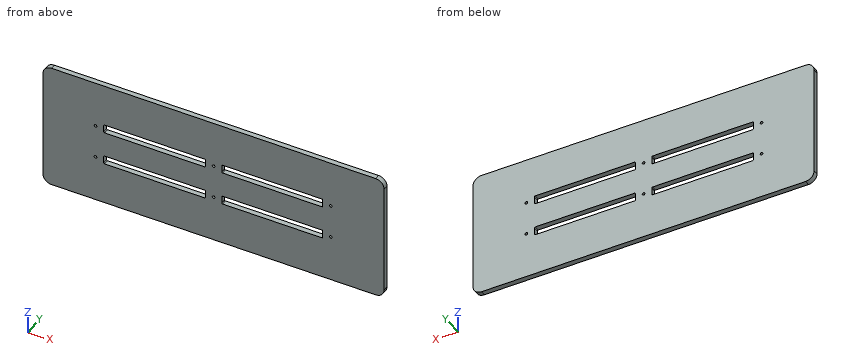
from build123d import *

# Parameters (mm, degrees)
IZIM1_W                     = 400
IZIM1_H                     = 150
IZIM1_W_2                   = 119.18
IZIM1_H_2                   = 10
IZIM1_W_3                   = 118.39
Y_KSEKLIK_EKSTR_ZYON1_DEPTH = 6
RADYUS1_R                   = 10
RADYUS2_R                   = 1
IZIM2_R                     = 1.575
KES_EKSTR_ZYON1_DEPTH       = 7


with BuildPart() as part:
    # Çizim1 → Yükseklik-Ekstrüzyon1 (new body)
    with BuildSketch(Plane(origin=(0, 0, 0), x_dir=(1, 0, 0), z_dir=(0, 1, 0))):
        Rectangle(IZIM1_W, IZIM1_H)
        with Locations((-69.19, 20)):
            Rectangle(IZIM1_W_2, IZIM1_H_2, mode=Mode.SUBTRACT)
        with Locations((68.795, 20)):
            Rectangle(IZIM1_W_3, IZIM1_H_2, mode=Mode.SUBTRACT)
        with Locations((68.795, -20)):
            Rectangle(IZIM1_W_3, IZIM1_H_2, mode=Mode.SUBTRACT)
        with Locations((-69.19, -20)):
            Rectangle(IZIM1_W_2, IZIM1_H_2, mode=Mode.SUBTRACT)
    extrude(amount=-Y_KSEKLIK_EKSTR_ZYON1_DEPTH)

    # Radyus1
    radyus1_edges = [part.edges().sort_by_distance(p)[0] for p in [
        (200, -3, 75),
        (-200, -3, 75),
        (-200, -3, -75),
        (200, -3, -75),
    ]]
    fillet(radyus1_edges, radius=RADYUS1_R)

    # Radyus2
    radyus2_edges = [part.edges().sort_by_distance(p)[0] for p in [
        (9.6, -3, -15),
        (9.6, -3, -25),
        (127.99, -3, -25),
        (127.99, -3, -15),
        (-9.6, -3, -25),
        (-9.6, -3, -15),
        (-128.78, -3, -15),
        (-128.78, -3, -25),
        (127.99, -3, 15),
        (127.99, -3, 25),
        (9.6, -3, 25),
        (9.6, -3, 15),
        (-9.6, -3, 15),
        (-9.6, -3, 25),
        (-128.78, -3, 25),
        (-128.78, -3, 15),
    ]]
    fillet(radyus2_edges, radius=RADYUS2_R)

    # Çizim2 → Kes-Ekstrüzyon1 (cut, through all)
    with BuildSketch(Plane.XZ.offset(6)):
        with Locations((-138.38, 20)):
            Circle(IZIM2_R)
        with Locations((-138.38, -20)):
            Circle(IZIM2_R)
        with Locations((0, -20)):
            Circle(IZIM2_R)
        with Locations((0, 20)):
            Circle(IZIM2_R)
        with Locations((137.59, 20)):
            Circle(IZIM2_R)
        with Locations((137.59, -20)):
            Circle(IZIM2_R)
    extrude(amount=-KES_EKSTR_ZYON1_DEPTH, mode=Mode.SUBTRACT)


solid = part.part
For this review, take the finished solid that the model builds, in its own axes (mm). Coordinates: 2 decimals unless noted, no trailing zeros. Write each question's results on one line, items separated by ' | '. Start each with the question number.
1) Wall thickness on L1, parallel to Z at x = 105, y = -5.1; L2, parallel to Z at x = 137.59, y = -4.45 (3 decimals): over which ranges is each line inside the solid? List them lowest first. Write a range as [from, to].
2) Insertion check: pin 1 (3 mm diameter, centred on x = 137.59, z = 20, fed in from -Y). The pin has a flat end and moves straight along its axis. Give the tip position at first contact, or say it passes through.
3) Consider section A-A (y = -2.35). Give the number of separate pieces and of enclosed holes in the cut face, plus the area to 3 significant figures.
Geometry says:
1) L1: [-75, -25], [-15, 15], [25, 75] | L2: [-75, -21.575], [-18.425, 18.425], [21.575, 75]
2) pin 1: through
3) separate pieces: 1 | enclosed holes: 10 | area: 55,100 mm^2
